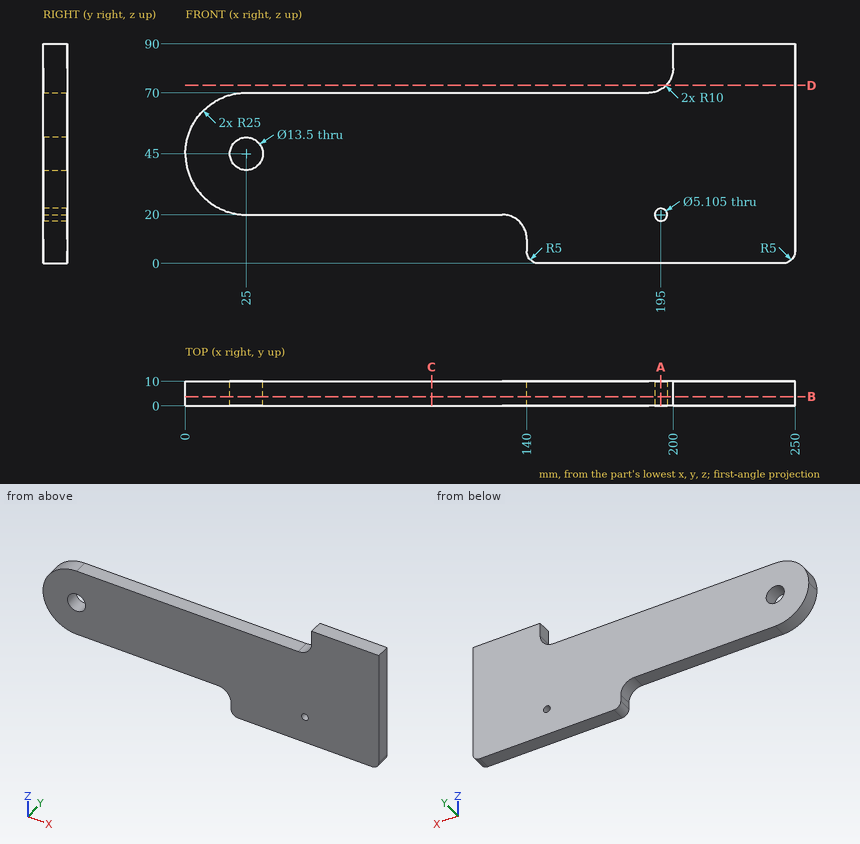
Design review of the part shown in the three views and the two pictorial views. Dimensions are in mm from the part's minimum x, y and z. Round coordinates to 2 decimals unless told otherwise and drop trailing zeros. Order: outer loops, then holes, each group sorted by start corner. A loop starts at its lowest first (then second) coordinate and runs counter-clockwise, first axis right, second up.
(1) Wall thickness on L1, parallel to X at y = 6, z = 45; L2, parallel to Z at x = 195, y = 7.5; L3, parallel to Z at x = 123, y = 5.75: over which ranges is each line inside the solid? List them lowest first.
Working result:
L1: x = 0 to 18.25, 31.75 to 250
L2: z = 0 to 17.45, 22.55 to 71.34
L3: z = 20 to 70
(2) Take a section at B-B, the plane y = 3.75. Count the separate pieces of the cut face and the enclosed holes in it, plus the area to 3 significant figures.
Working result:
separate pieces: 1
enclosed holes: 2
area: 15,300 mm2
(3) Take a section at C-C, the plane x = 101. State the section outline as (y, z) points.
Working result:
outline: (0, 20) - (10, 20) - (10, 70) - (0, 70) - close
(4) Take a section at D-D, the plane z = 73. State the section outline as (x, y) points.
Working result:
outline: (197.14, 0) - (250, 0) - (250, 10) - (197.14, 10) - close
(5) For P1, Ø2, axis at y = 2, z = 21.5, coming from the -X side (1 decimal); P2, Ø6, axis at y = 5, z = 11.5, coming from the -X side; P3, Ø1.5, axis at x = 37.5, y = 6, coming from the +Z side, all flat-tipped, find the tip position at first contact; note any pin that passes through.
Working result:
P1: stops at x = 14.1
P2: stops at x = 138.93
P3: stops at z = 70
(6) Take a section at A-A, the plane x = 195. State the section outline as (y, z) points, plus the area to 3 significant figures.
Working result:
outline: (0, 0) - (10, 0) - (10, 17.45) - (0, 17.45) - close; (0, 22.55) - (10, 22.55) - (10, 71.34) - (0, 71.34) - close
area: 662 mm2
